Geometry check sheet. Reference: the model listing, model coordinates, mm. Coordinates: 2 decimals unless noted, no trailing zeros. Write each loop counter-clockwise with the first axis right and the second up, starting at its lowest first coordinate (ties: lowest second). Pieces come first, ordered by that corner, then holes. Notation, with made-up numbers: (-35, 54.25) -> (-21, 54.25) arc R15 cw to (-21, 75.25) -> close; hole circle Ø9 at (44.5, 34.25). An arc over 180 degrees is marked (long way). One line per question, with ' | ' between items.
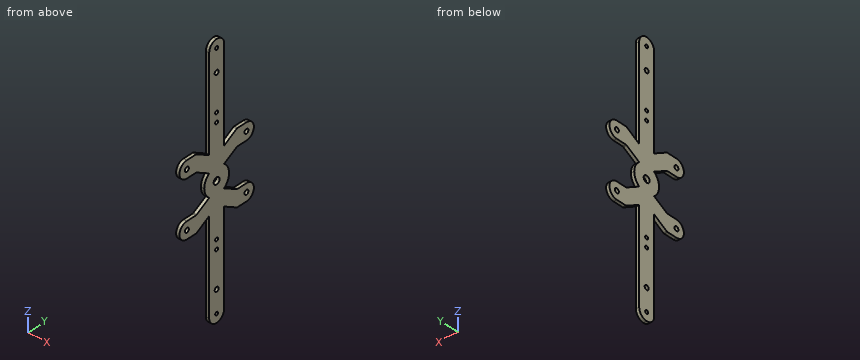
```python
from build123d import *

# Parameters (mm, degrees)
SKETCH1_W               = 250
SKETCH1_H               = 90
BOSS_EXTRUDE1_DEPTH     = 3
SKETCH2_R               = 3
SKETCH2_R_2             = 1.5
SKETCH2_R_3             = 2
CUT_EXTRUDE1_DEPTH      = 4
SKETCH3_R               = 2
CUT_EXTRUDE2_DEPTH      = 4
CUT_EXTRUDE3_DEPTH      = 4
MIRROR2_COPY_1_SKETCH_R = 2
MIRROR2_COPY_1_DEPTH    = 4
MIRROR2_COPY_2_DEPTH    = 4
FILLET2_R               = 2


with BuildPart() as part:
    # Sketch1 → Boss-Extrude1 (new body)
    with BuildSketch(Plane(origin=(0, 0, 0), x_dir=(0, 0, -1), z_dir=(1, 0, 0))):
        Rectangle(SKETCH1_W, SKETCH1_H)
    extrude(amount=BOSS_EXTRUDE1_DEPTH)

    # Sketch2 → Cut-Extrude1 (cut, through all)
    with BuildSketch(Plane(origin=(3, 0, 0), x_dir=(0, 0, -1), z_dir=(1, 0, 0))):
        Circle(SKETCH2_R)
        with Locations((-48, 0)):
            Circle(SKETCH2_R_2)
        with Locations((-89, 0)):
            Circle(SKETCH2_R_3)
        with Locations((-109, 0)):
            Circle(SKETCH2_R_2)
        with Locations((-56.18, 0)):
            Circle(SKETCH2_R_2)
    cut_extrude1 = extrude(amount=-CUT_EXTRUDE1_DEPTH, mode=Mode.SUBTRACT)

    # Sketch3 → Cut-Extrude2 (cut, through all)
    with BuildSketch(Plane(origin=(3, 0, 0), x_dir=(0, 0, -1), z_dir=(1, 0, 0))):
        with Locations((-25, 30)):
            Circle(SKETCH3_R)
    cut_extrude2 = extrude(amount=-CUT_EXTRUDE2_DEPTH, mode=Mode.SUBTRACT)

    # Sketch4 → Cut-Extrude3 (cut, through all)
    with BuildSketch(Plane(origin=(3, 0, 0), x_dir=(0, 0, -1), z_dir=(1, 0, 0))):
        with BuildLine():
            Line((-125, 1.99556796), (-125, 45))
            Line((-125, 45), (0, 45))
            Line((0, 45), (0, 12.5))
            ThreePointArc((0, 12.5), (-5.582012149, 11.184415066), (-9.989046524, 7.514582459))
            Line((-9.989046524, 7.514582459), (-17.5, 20.523935493))
            Line((-17.5, 20.523935493), (-17.5, 30))
            ThreePointArc((-17.5, 30), (-25, 37.5), (-32.5, 30))
            Line((-32.5, 30), (-32.5, 20.523935493))
            Line((-32.5, 20.523935493), (-24.989046524, 7.514582459))
            Line((-24.989046524, 7.514582459), (-109, 7.514582459))
            ThreePointArc((-109, 7.514582459), (-114.313612215, 5.313612215), (-116.514582459, 0))
            Line((-116.514582459, 0), (-125, 0))
            Line((-125, 0), (-125, 1.99556796))
        make_face()
    cut_extrude3 = extrude(amount=-CUT_EXTRUDE3_DEPTH, mode=Mode.SUBTRACT)

    # Mirror1: Cut-Extrude2, Cut-Extrude3 across plane
    add(cut_extrude2.mirror(Plane.ZX), mode=Mode.SUBTRACT)
    add(cut_extrude3.mirror(Plane.ZX), mode=Mode.SUBTRACT)

    # Mirror2: Cut-Extrude1, Cut-Extrude2, Cut-Extrude3 across plane
    add(cut_extrude1.mirror(Plane.XY), mode=Mode.SUBTRACT)
    add(cut_extrude2.mirror(Plane.XY), mode=Mode.SUBTRACT)
    add(cut_extrude3.mirror(Plane.XY), mode=Mode.SUBTRACT)

    # Mirror2 copy 1 sketch → Mirror2 copy 1 (cut, through all)
    with BuildSketch(Plane(origin=(3, 0, 0), x_dir=(0, 0, 1), z_dir=(1, 0, 0))):
        with Locations((-25, 30)):
            Circle(MIRROR2_COPY_1_SKETCH_R)
    extrude(amount=-MIRROR2_COPY_1_DEPTH, mode=Mode.SUBTRACT)

    # Mirror2 copy 2 sketch → Mirror2 copy 2 (cut, through all)
    with BuildSketch(Plane(origin=(3, 0, 0), x_dir=(0, 0, 1), z_dir=(1, 0, 0))):
        with BuildLine():
            Line((-125, 1.99556796), (-125, 45))
            Line((-125, 45), (0, 45))
            Line((0, 45), (0, 12.5))
            ThreePointArc((0, 12.5), (-5.582012149, 11.184415066), (-9.989046524, 7.514582459))
            Line((-9.989046524, 7.514582459), (-17.5, 20.523935493))
            Line((-17.5, 20.523935493), (-17.5, 30))
            ThreePointArc((-17.5, 30), (-25, 37.5), (-32.5, 30))
            Line((-32.5, 30), (-32.5, 20.523935493))
            Line((-32.5, 20.523935493), (-24.989046524, 7.514582459))
            Line((-24.989046524, 7.514582459), (-109, 7.514582459))
            ThreePointArc((-109, 7.514582459), (-114.313612215, 5.313612215), (-116.514582459, 0))
            Line((-116.514582459, 0), (-125, 0))
            Line((-125, 0), (-125, 1.99556796))
        make_face()
    extrude(amount=-MIRROR2_COPY_2_DEPTH, mode=Mode.SUBTRACT)

    # Fillet2
    fillet2_edges = [part.edges().sort_by_distance(p)[0] for p in [
        (1.5, -20.523935493, -32.5),
        (1.5, -20.523935493, -17.5),
        (1.5, 20.523935493, -17.5),
        (1.5, 20.523935493, -32.5),
        (1.5, 20.523935493, 32.5),
        (1.5, 20.523935493, 17.5),
        (1.5, -20.523935493, 17.5),
        (1.5, -20.523935493, 32.5),
    ]]
    fillet(fillet2_edges, radius=FILLET2_R)


solid = part.part
```
(1) Cross-section at C-C (x = 2.2). Count the separate pieces of the cut face and the enclosed holes in it, plus the area to 3 significant figures.
Answers below:
separate pieces: 1 | enclosed holes: 13 | area: 5,150 mm²
(2) Cross-section at D-D (z = 13). Record the cut outline in (x, y).
Answers below:
outline: (0, -12.73) -> (3, -12.73) -> (3, 12.73) -> (0, 12.73) -> close
(3) Cross-section at B-B (y = -23.5). Record the cut outline in (x, z), plus the area to 3 significant figures.
Answers below:
outline: (0, -32.5) -> (3, -32.5) -> (3, -17.5) -> (0, -17.5) -> close; (0, 17.5) -> (3, 17.5) -> (3, 32.5) -> (0, 32.5) -> close | area: 90.0 mm²
(4) Depth check by flat-ended pin: P1, Ø0.9, axis at x = 1.5, y = -26, coming from the -Z side; P2, Ø1.5, axis at x = 0.5, y = 4, coming from the -Z side; P3, Ø0.9, axis at x = 1, z = 47, coming from the +Y side. Enter the tip coordinate at first touch or a pass-through.
Answers below:
P1: stops at z = -32.5 | P2: stops at z = -115.78 | P3: stops at y = 7.51
(5) Material ranges on line 1 (Z direction, x = 1.75, y = -30); line 2 (Y direction, x = 1.15, z = -48); line 3 (Z direction, x = 1.4, y = -21), recorded low to high.
Answers below:
line 1: z = -32.5 to -27, -23 to -17.5, 17.5 to 23, 27 to 32.5 | line 2: y = -7.51 to -1.5, 1.5 to 7.51 | line 3: z = -32.5 to -17.5, 17.5 to 32.5
(6) Cross-section at A-A (z = -89). Record the cut outline in (x, y), plus the area to 3 significant figures.
Answers below:
outline: (0, -7.51) -> (3, -7.51) -> (3, -2) -> (0, -2) -> close; (0, 2) -> (3, 2) -> (3, 7.51) -> (0, 7.51) -> close | area: 33.1 mm²
